from build123d import *

# Parameters (mm, degrees)
PAD_DEPTH       = 5
PAD001_DEPTH    = 46.52
SKETCH002_W     = 5
SKETCH002_H     = 5
PAD002_DEPTH    = 46.52
PAD003_DEPTH    = 5
SKETCH004_R     = 6
SKETCH004_R_2   = 1.2
POCKET_DEPTH    = 5
SKETCH005_R     = 6
SKETCH005_R_2   = 1.2
POCKET001_DEPTH = 75.732575
FILLET_R        = 14
FILLET001_R     = 15
FILLET002_R     = 15
FILLET003_R     = 15
FILLET004_R     = 10
FILLET005_R     = 10


with BuildPart() as part:
    # Sketch → Pad (new body)
    with BuildSketch(Plane.XZ):
        Polygon((0, 0), (37.553362, -6.621671), (50.053362, 15.028964), (5, 46.575668), (0, 46.575668), align=None)
    extrude(amount=PAD_DEPTH)

    # Sketch001 → Pad001 (new body)
    with BuildSketch(Plane(origin=(0, 0, 46.575668), x_dir=(-1, 0, 0), z_dir=(0, 0, 1))):
        Polygon((0, 5), (8.829476, 0.305284), (8.829476, -66.03686), (0, -70.731575), (0, -65.731575), (4.96369, -62.865788), (4.96369, -2.865788), (0, 0), align=None)
    extrude(amount=-PAD001_DEPTH)

    # Sketch002 → Pad002 (new body)
    with BuildSketch(Plane(origin=(0, 0, 46.575668), x_dir=(-1, 0, 0), z_dir=(0, 0, 1))):
        with Locations((-2.5, -68.231575)):
            Rectangle(SKETCH002_W, SKETCH002_H)
    extrude(amount=-PAD002_DEPTH)

    # Sketch003 → Pad003 (new body)
    with BuildSketch(Plane(origin=(0, 70.731575, 0), x_dir=(1, 0, 0), z_dir=(0, 1, 0))):
        Polygon((5, -0.055668), (5, -46.575668), (50.368156, -15.48338), (37.651222, 6.040551), align=None)
    extrude(amount=-PAD003_DEPTH)

    # Sketch004 → Pocket (cut)
    with BuildSketch(Plane(origin=(-8.829476, 0, 0), x_dir=(0, 0, -1), z_dir=(-1, 0, 0))):
        with Locations((-23.287834, -32.865788)):
            Circle(SKETCH004_R)
        with Locations((-23.287834, -21.865788)):
            Circle(SKETCH004_R_2)
        with Locations((-23.287834, -17.865788)):
            Circle(SKETCH004_R_2)
        with Locations((-23.287834, -43.865788)):
            Circle(SKETCH004_R_2)
        with Locations((-23.287834, -47.865788)):
            Circle(SKETCH004_R_2)
    extrude(amount=-POCKET_DEPTH, mode=Mode.SUBTRACT)

    # Sketch005 → Pocket001 (cut, through all)
    with BuildSketch(Plane.XZ.offset(5)):
        with Locations((13.106433, 21.398445)):
            Circle(SKETCH005_R)
        with Locations((22.117105, 15.089104)):
            Circle(SKETCH005_R_2)
        with Locations((25.393713, 12.794799)):
            Circle(SKETCH005_R_2)
    extrude(amount=-POCKET001_DEPTH, mode=Mode.SUBTRACT)

    # Fillet
    fillet_edges = [part.edges().sort_by_distance(p)[0] for p in [
        (50.053362, -2.5, 15.028964),
    ]]
    fillet(fillet_edges, radius=FILLET_R)

    # Fillet001
    fillet001_edges = [part.edges().sort_by_distance(p)[0] for p in [
        (37.553362, -2.5, -6.621671),
    ]]
    fillet(fillet001_edges, radius=FILLET001_R)

    # Fillet002
    fillet002_edges = [part.edges().sort_by_distance(p)[0] for p in [
        (50.368156, 68.231575, 15.48338),
    ]]
    fillet(fillet002_edges, radius=FILLET002_R)

    # Fillet003
    fillet003_edges = [part.edges().sort_by_distance(p)[0] for p in [
        (37.651222, 68.231575, -6.040551),
    ]]
    fillet(fillet003_edges, radius=FILLET003_R)

    # Fillet004
    fillet004_edges = [part.edges().sort_by_distance(p)[0] for p in [
        (5, -2.5, 46.575668),
    ]]
    fillet(fillet004_edges, radius=FILLET004_R)

    # Fillet005
    fillet005_edges = [part.edges().sort_by_distance(p)[0] for p in [
        (5, 68.231575, 46.575668),
    ]]
    fillet(fillet005_edges, radius=FILLET005_R)


solid = part.part
Model file for the job. Use its own axes, mm. A direction names the side the tool comes from. Round coordinates to 2 decimals unless told otherwise and drop trailing zeros. Order: outer loops, then holes, each group sorted by start corner. A loop starts at its lowest first (then second) coordinate and runs counter-clockwise, first axis right, second up.
(1) Band-saw the part on B-B (z = -2). List the corners of the cut face in (x, y).
(2) Band-saw the part on D-D (y = 9). List the corners of the cut face in (x, z), then the cut area to 3 significant figures.
(3) Band-saw the part on C-C (z = 32.5). List the corners of the cut face in (x, y), then the cut area to 3 significant figures.
(4) 3-axis set-ups, long thin cutter, end or side, ignore diameter. For faces 3 (the face through (-4.964, 26.6, 23.6)), 4 (the face through (45.15, -2.54, 14.09)), 5 (the face through (23.79, -2.46, 33.42)): which of +Z, -Z, +X, -X, +Y, -Y reach the whole face in a straight line?
(5) Band-saw the part on A-A (x = 13.5). List the corners of the cut face in (y, z), then the cut area to 3 significant figures.
(6) Pull direction Y, two halves, no side cores. Call faces 1 (the face through (12.33, -2.54, 27.35)), 2 (the face through (17, 0, 15)): released by +Y, released by -Y, zero draft, split by the parting line, or undercut.
(7) Drill centre lines: line 1 (Y direction, x = 7, z = 36.5); line 2 (X direction, y = 47, z = 37); line 3 (Y direction, x = -1.5, z = 37). Where is each one in solid material? Low to high.
(8) Pin check, flat tips, straight feed: pin 1 (2 mm diameter, centred on y = 17.87, z = 23.29, fed in from -X); pin 2 (3 mm diameter, centred on x = 25.39, z = 12.79, fed in from +Y); pin 3 (8 mm diameter, centred on y = 22.5, z = 29.5, fed in from +X). Stop position of each tip, or through.
Verdict:
1. outline: (11.34, -5) - (38.85, -5) - (38.85, 0) - (11.34, 0) - close; (16.01, 65.73) - (38.17, 65.73) - (38.17, 70.73) - (16.01, 70.73) - close
2. outline: (-8.83, 0.06) - (-4.96, 0.06) - (-4.96, 46.58) - (-8.83, 46.58) - close
2. area: 180 mm2
3. outline: (-8.83, -0.31) - (0, -5) - (25.1, -5) - (25.1, 0) - (0, 0) - (-4.96, 2.87) - (-4.96, 62.87) - (0, 65.73) - (25.54, 65.73) - (25.54, 70.73) - (0, 70.73) - (-8.83, 66.04) - close
3. area: 568 mm2
4. face 3: +Z, -Z, +X
4. face 4: +X, -Y
4. face 5: +Z, +X, -Y
5. outline: (-5, -2.38) - (0, -2.38) - (0, 15.41) - (-5, 15.41) - close; (-5, 27.39) - (0, 27.39) - (0, 40.62) - (-5, 40.62) - close; (65.73, -1.53) - (70.73, -1.53) - (70.73, 15.41) - (65.73, 15.41) - close; (65.73, 27.39) - (70.73, 27.39) - (70.73, 40.75) - (65.73, 40.75) - close
5. area: 307 mm2
6. face 1: zero draft
6. face 2: undercut
7. line 1: y = -5 to 0, 65.73 to 70.73
7. line 2: x = -8.83 to -4.96
7. line 3: y = -4.2 to 0.87, 64.87 to 69.93
8. pin 1: passes through
8. pin 2: stops at y = 70.73
8. pin 3: stops at x = -4.96
